Input: dimensioned drawing with shaded views. Units: mm. Origin: part minimum x, y, z. Coordinates: 2 decimals unless noted, no trailing zeros. Loops run counter-clockwise (first coordinate to the right, second up) from the corner with the lowest first, then second, coordinate; pieces in that order, holes last.
Item 1: Section A-A on y = 40. Return loops of the section in (x, z), and give its area (3 significant figures).
Item 2: Ray query, line 1 along Y through (x, z) = (80, 1.95); line 2 along Y through (x, z) = (263, 3.35). Return the intervals inside material, ascending.
Item 3: Section D-D on x = 165.5. Return loops of the section in (y, z), and give its area (3 significant figures).
Item 4: Section B-B on z = 2.8. Return loops of the section in (x, y).
Item 5: Section C-C on x = 80. Return loops of the section in (y, z).
Item 6: Contact query for flat-ended pins moving along their axis: P1, Ø6.5, axis at x = 80, y = 40, coming from the +Z side; P2, Ø3, axis at y = 203, z = 4.5, coming from the +X side; P3, Ø3, axis at x = 168, z = 2.5, coming from the +Y side. Output: stop coordinate, or through.
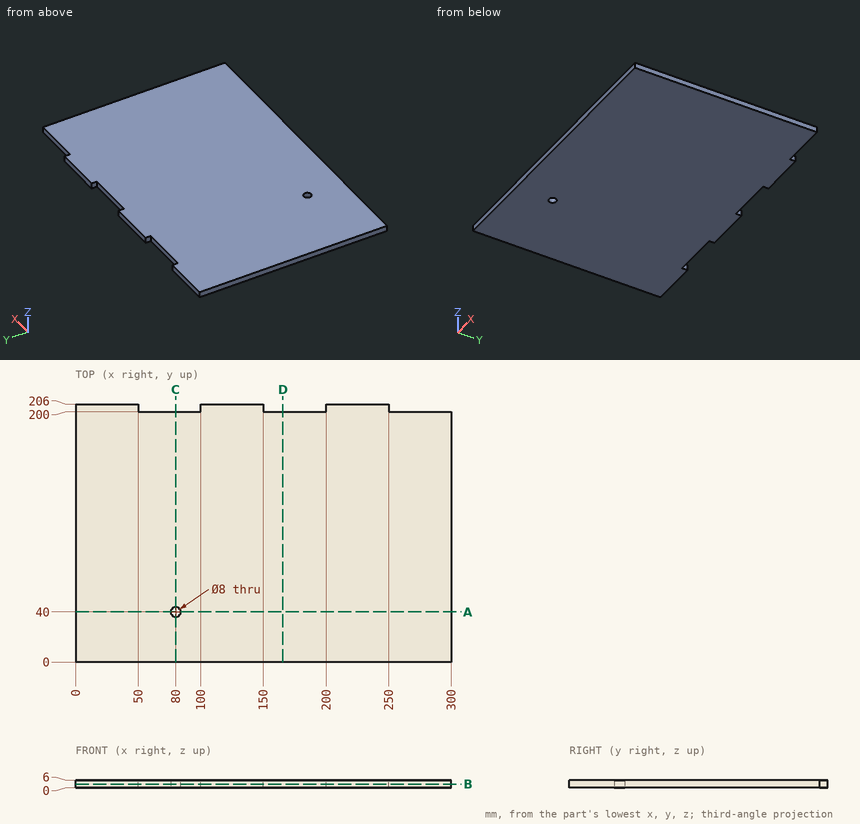
Results found:
1. outline: (0, 0) - (76, 0) - (76, 6) - (0, 6) - close; (84, 0) - (300, 0) - (300, 6) - (84, 6) - close
1. area: 1,750 mm2
2. line 1: y = 0 to 36, 44 to 200
2. line 2: y = 0 to 200
3. outline: (0, 0) - (200, 0) - (200, 6) - (0, 6) - close
3. area: 1,200 mm2
4. outline: (0, 0) - (300, 0) - (300, 200) - (250, 200) - (250, 206) - (200, 206) - (200, 200) - (150, 200) - (150, 206) - (100, 206) - (100, 200) - (50, 200) - (50, 206) - (0, 206) - close; hole circle Ø8 at (80, 40)
5. outline: (0, 0) - (36, 0) - (36, 6) - (0, 6) - close; (44, 0) - (200, 0) - (200, 6) - (44, 6) - close
6. P1: passes through
6. P2: stops at x = 250
6. P3: stops at y = 200
